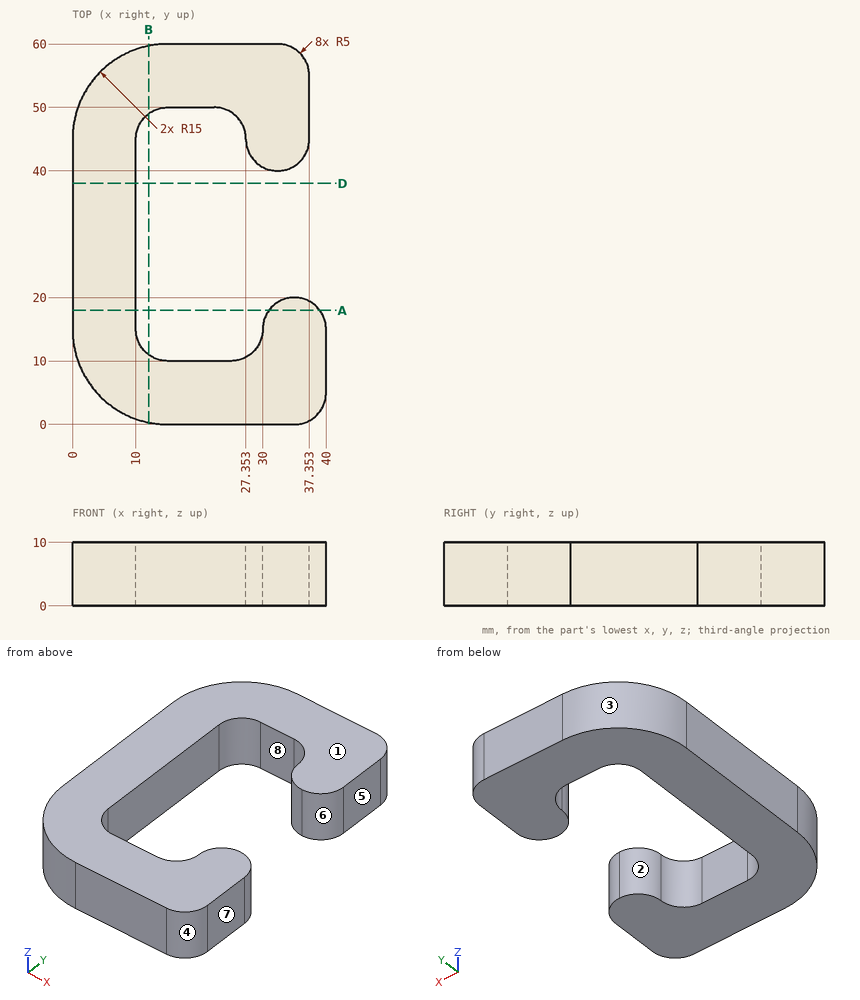
Here's the drawing with two shaded views (mm, measured from the low corner). I have some questions. A direction names the side the tool comes from. Coordinates: 2 decimals unless noted, no trailing zeros. Order: outer loops, then holes, each group sorted by start corner. A loop starts at its lowest first (then second) coordinate and runs counter-clockwise, first axis right, second up. Notation, with made-up numbers: (-30.5, 7.25) - (-0.5, 7.25) arc R17 ccw to (-0.5, 11.25) - close; hole circle Ø10 at (42.5, 13.5). An arc over 180 degrees is marked (long way). Use CSV: the item, a comma, the result in double quotes. Start each with the question number.
1. Suppose I cut it at D-D on y = 38. List the corners of the cut face in (x, z) for me.
2. For the marked faces 4, 5, 6, 7 and 8, which set-ups out of +Z, -Z, +X, -X, +Y, -Y let a thin tool reach every point of the face, with its end or its side?
3. Please list where these lines run through material, in increasing order: line 1 (Y direction, x = 20.5, z = 6); line 2 (Y direction, x = 24, z = 8.25); line 3 (X direction, y = 11.5, z = 9.5). Write a range as from..to.
4. If we mould it in two halves opening along Y, with no side actions, what happens to the marked faces 1, 2 and 3? For each: +Y half, -Y half, draft (parallel to the pull), parting line (faces both ways), or undercut.
5. Suppose I cut it at A-A on y = 18. List the corners of the cut face in (x, z) for me.
6. Suppose I cut it at B-B on x = 12. List the corners of the cut face in (y, z) for me, then the cut area to 3 significant figures.
7. I'm going to push flat-ended pins straight in: pin 1 (1 mm diameter, centred on y = 37, z = 2, fed in from +X); pin 2 (3 mm diameter, centred on x = 35.5, z = 4.5, fed in from +Y); pin 3 (1.5 mm diameter, centred on x = 9.5, z = 2, fed in from -Y). Where does each tip first touch, or does it pass through?
Output:
1,outline,"(0, 0) - (10, 0) - (10, 10) - (0, 10) - close"
2,face 4,"+Z, -Z, +X, -Y"
2,face 5,"+Z, -Z, +X, +Y"
2,face 6,"+Z, -Z, +X"
2,face 7,"+Z, -Z, +X, +Y, -Y"
2,face 8,"+Z, -Z"
3,line 1,"y = 0..10, 50..60"
3,line 2,"y = 0..10, 49.72..60"
3,line 3,"x = 0.41..11.43, 28.57..40"
4,face 1,"draft"
4,face 2,"undercut"
4,face 3,"+Y half"
5,outline,"(0, 0) - (10, 0) - (10, 10) - (0, 10) - close; (31, 0) - (39, 0) - (39, 10) - (31, 10) - close"
6,outline,"(0.3, 0) - (11, 0) - (11, 10) - (0.3, 10) - close; (49, 0) - (59.7, 0) - (59.7, 10) - (49, 10) - close"
6,area,"214 mm2"
7,pin 1,"stops at x = 10"
7,pin 2,"stops at y = 59.72"
7,pin 3,"stops at y = 0.77"
